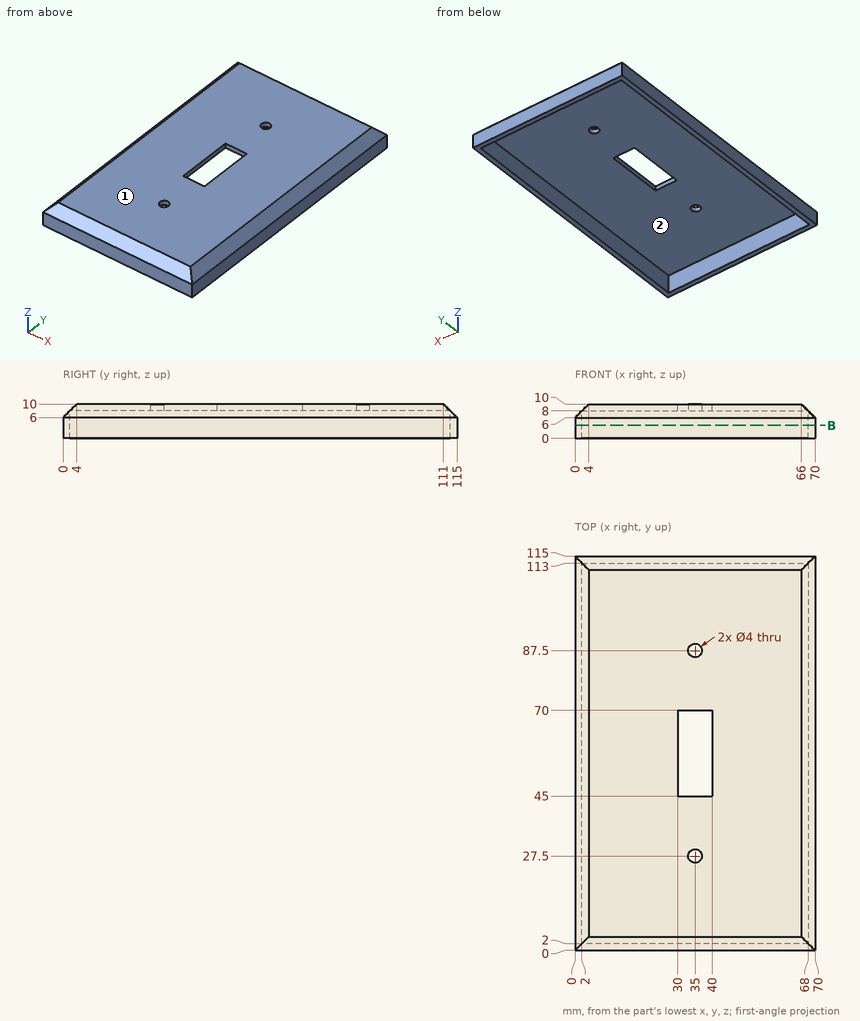
Source: three-view drawing plus pictorial views. Frame: mm from the lowest corner of the part. Give positions to 0.01 mm unless a question says otherwise; leave off trailing zeros. Write each loop counter-clockwise with the first axis right and the second up, starting at its lowest first coordinate (ties: lowest second). Pieces come first, ordered by that corner, then holes. Notation, with made-up numbers: (11, 20.5) -> (56, 20.5) arc R37 cw to (56, 58.5) -> close; hole circle Ø6 at (66, -4). An arc over 180 degrees is marked (long way). Write item = value, one per line.
Q1. Line query: line 1 (X direction, y = 25.5, z = 2); line 2 (Y direction, x = 42, z = 4); line 3 (X direction, y = 87.5, z = 8.4). Output: solid intervals per line, ascending. Write a range as from..to.
Here are the results:
line_1 = 0..2, 68..70
line_2 = 0..2, 113..115
line_3 = 2.4..33, 37..67.6
Q2. Cut plane B-B on z = 3.75. Return loops of the section in (x, y).
Here are the results:
outline = (0, 0) -> (70, 0) -> (70, 115) -> (0, 115) -> close; hole (2, 2) -> (68, 2) -> (68, 113) -> (2, 113) -> close
Q3. First-contact query: pin 1 (0.6 mm diameter, centred on y = 53.5, z = 9.5, fed in from -X); pin 2 (1.6 mm diameter, centred on y = 62, z = 9.5, fed in from +X); pin 3 (2 mm diameter, centred on x = 36.5, z = 8.5, fed in from +Y); pin 4 (2.5 mm diameter, centred on x = 35, y = 27.5, fed in from +Z). Flat tips, straight axial feed; report the tip coordinate or a pass-through.
Here are the results:
pin_1 = 3.2
pin_2 = 67.3
pin_3 = 113.5
pin_4 = through
Q4. Mould query, pull axis X, two halves, no side actions, for the marked faces 1 and 2. Classes: +X half, -X half, draft (parallel to the pull), parting line (faces both ways), or undercut.
Here are the results:
face_1 = draft
face_2 = undercut
